Input: dimensioned drawing with shaded views. Units: mm. Origin: part minimum x, y, z. Round coordinates to 2 decimals unless told otherwise and drop trailing zeros. Loops run counter-clockwise (first coordinate to the right, second up) from the corner with the lowest first, then second, coordinate; pieces in that order, holes last. Notation, with made-up numbers: (-1.5, 8) - (33.5, 8) arc R19 ccw to (33.5, 33) - close; hole circle Ø5 at (-8.75, -30.5). An arc over 180 degrees is marked (long way). Write each question's results on one line, items separated by ' | '.
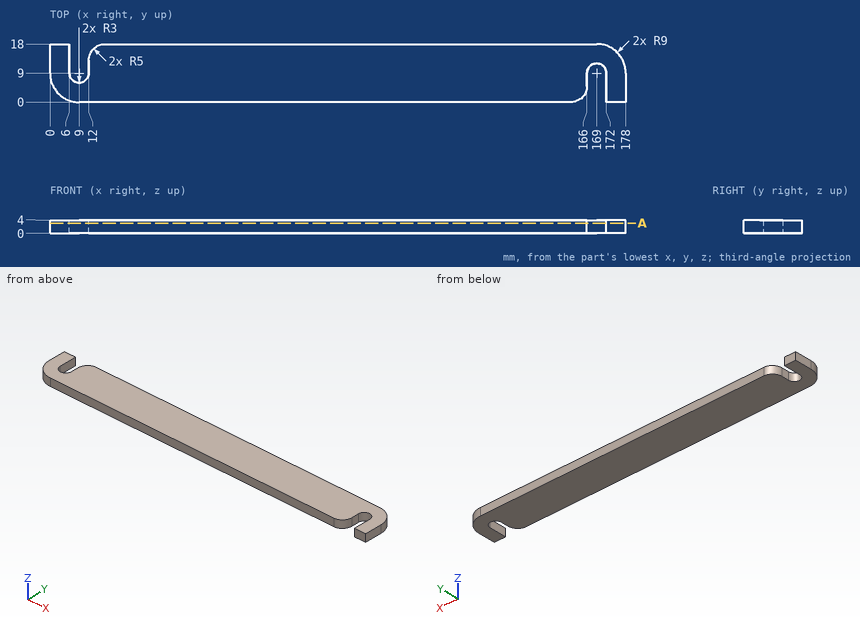
1. Section query A-A, the plane z = 3.1. Output: boundary loops of the cut face in (x, y).
Answer:
outline: (0, 9) arc R9 ccw to (9, 0) - (161, 0) arc R5 ccw to (166, 5) - (166, 9) arc R3 cw to (172, 9) - (172, 0) - (178, 0) - (178, 9) arc R9 ccw to (169, 18) - (17, 18) arc R5 ccw to (12, 13) - (12, 9) arc R3 cw to (6, 9) - (6, 18) - (0, 18) - close
2. Contact query for flat-ended pins moving along their axis: pin 1 (8 mm diameter, centred on x = 148.5, y = 9, fed in from -Z); pin 2 (1.5 mm diameter, centred on y = 12.5, z = 2, fed in from +X); pin 3 (1.2 mm diameter, centred on y = 14.5, z = 1.5, fed in from +X). Output: stop coordinate, or through.
Answer:
pin 1: z = 0 | pin 2: x = 177.57 | pin 3: x = 176.55
3. Line query: line 1 (X direction, y = 8.75, z = 2.8); line 2 (X direction, y = 7.5, z = 2.5); line 3 (Y direction, x = 169, z = 2.4). Output: solid intervals per line, ascending. Write a range as [from, to].
Answer:
line 1: [0, 6.01], [11.99, 166], [172, 178] | line 2: [0.13, 6.4], [11.6, 166], [172, 178] | line 3: [12, 18]
